Read the model definition and answer for the solid it produces. Units are mm, in the model's axes. A direction names the side the tool comes from. Give positions to 0.01 mm unless a question says otherwise; leave off trailing zeros. Loops run counter-clockwise (first coordinate to the right, second up) from the corner with the lowest first, then second, coordinate; pieces in that order, holes last. Notation, with made-up numbers: (-36.75, -24) -> (-31.75, -24) arc R29 ccw to (-31.75, 2) -> close; hole circle Ø6 at (41, 46.25). An arc over 180 degrees is marked (long way). One line per item, written item: value. Start each with the question number.
from build123d import *

# Parameters (mm, degrees)
F3_DEPTH = 13.97


with BuildPart() as f1:
    # F0 (on Front) → F1 (revolve)
    with BuildSketch(Plane.XZ):
        with BuildLine():
            Line((7.876178, -20.195216), (8.228687, 0))
            Line((8.228687, 0), (7.876178, 20.195216))
            ThreePointArc((7.876178, 20.195216), (7.838213, 20.283583), (7.749197, 20.32))
            Line((7.749197, 20.32), (6.347803, 20.32))
            ThreePointArc((6.347803, 20.32), (6.258787, 20.283583), (6.220822, 20.195216))
            Line((6.220822, 20.195216), (5.868313, 0))
            Line((5.868313, 0), (7.041552, -20.200364))
            ThreePointArc((7.041552, -20.200364), (7.081178, -20.285369), (7.168338, -20.32))
            Line((7.168338, -20.32), (7.749197, -20.32))
            ThreePointArc((7.749197, -20.32), (7.838213, -20.283583), (7.876178, -20.195216))
        make_face()
    revolve(axis=Axis((0, 0, 5.243593), (0, 0, -1)))

    # F2 (on Top) → F3 (join, symmetric)
    with BuildSketch(Plane.XY):
        with BuildLine():
            Line((-2.459506, 0.112758), (1.096672, 6.948127))
            ThreePointArc((1.096672, 6.948127), (0.550133, 7.015935), (0, 7.041552))
            Line((0, 7.041552), (-2.903674, 0.532035))
            Line((-2.903674, 0.532035), (-2.959069, 0.407848))
            ThreePointArc((-2.959069, 0.407848), (-2.841238, 0.036922), (-2.459506, 0.112758))
        make_face()
        with BuildLine():
            ThreePointArc((5.486935, -4.655437), (5.818928, -4.216025), (6.116179, -3.752404))
            Line((6.116179, -3.752404), (1.930609, 2.01701))
            Line((1.930609, 2.01701), (1.850757, 2.127077))
            ThreePointArc((1.850757, 2.127077), (1.470611, 2.210495), (1.345421, 1.841988))
            Line((1.345421, 1.841988), (5.486935, -4.655437))
        make_face()
        with BuildLine():
            Line((0.940514, -2.31779), (-6.757178, -2.655735))
            ThreePointArc((-6.757178, -2.655735), (-6.542632, -3.162955), (-6.28975, -3.652192))
            Line((-6.28975, -3.652192), (0.799493, -2.912089))
            Line((0.799493, -2.912089), (0.93474, -2.897969))
            ThreePointArc((0.93474, -2.897969), (1.197055, -2.610462), (0.940514, -2.31779))
        make_face()
    extrude(amount=F3_DEPTH, both=True)

    # F4 (on Front) → F5 (revolve, cut)
    with BuildSketch(Plane.XZ):
        Polygon((6.11216, 13.97), (0, 13.97), (0, 7.85784), align=None)
        Polygon((0, -7.290308), (0, -13.97), (6.679692, -13.97), align=None)
    revolve(axis=Axis((0, 0, 5.243593), (0, 0, -1)), mode=Mode.SUBTRACT)


solid = f1.part
Item 1: Section C-C, the plane z = 8.5 is taken. Determine the outline of the cut face in (x, y).
Item 2: For faces 4 (the conical face through (-2.26, -2.93, -10.99)), 5 (the flat face through (-4.6, 5.7, -20.32)), 6 (the conical face through (-1.93, -2.97, 11.4)), determine the directions among +Z, -Z, +X, -X, +Y, -Y from which every point of the face is accessible in a straight line to the end or side of a thin tool.
Item 3: Consider L1, parallel to Y at x = 1, z = -1; L2, parallel to X at y = 4.75, z = -1; L3, parallel to Y at x = -4.5, z = -9. Determine where each line is inside the solid, lowest interval first. Write a range as [from, to].
Item 4: Section A-A, the plane z = -1 is taken. Determine the outline of the cut face in (x, y), plus the area to 3 significant figures.
Item 5: Section B-B, the plane y = 4 is taken. State how many separate pieces and enclosed holes the cut face has, plus the area to 3 significant figures.
Item 6: Determine the mould class of faces 1 (the conical face through (-1.745, 7.859, 10.239)), 2 (the conical face through (3.211, -0.409, 11.094)), 3 (the flat face through (-3, 6, 20.32)) for opening direction Y: pulls with the +Y half, pulls with the -Y half, needs draft (parallel to the pull), parting line crosses it, or undercut.
Item 7: Flat-ended cylindrical pins translate along their axes: pin 1 (3 mm diameter, centred on x = 1, z = 1, fed in from -Y); pin 2 (6 mm diameter, centred on y = -4.5, z = -8, fed in from -X); pin 3 (4 mm diameter, centred on y = 0, z = 3, fed in from -X); pin 4 (6 mm diameter, centred on x = 5.5, z = -1.5, fed in from -Y). Find the tip coordinate at first contact, or state that the pin passes through.
Computed values:
1. outline: circle Ø16.16 at (0, 0); hole (-5.43, -2.6) -> (0.94, -2.32) arc R0.29 cw to (0.93, -2.9) -> (0.8, -2.91) -> (-4.89, -3.51) arc R6.02 ccw to (4.82, -3.6) -> (1.35, 1.84) arc R0.29 cw to (1.85, 2.13) -> (1.93, 2.02) -> (5.37, -2.72) arc R6.02 ccw to (0.6, 5.99) -> (-2.46, 0.11) arc R0.29 cw to (-2.96, 0.41) -> (-2.9, 0.53) -> (-0.47, 6) arc R6.02 ccw to start
2. face 4: -Z
2. face 5: -Z, +X, -X, +Y, -Y
2. face 6: +Z
3. L1: [-8.15, -5.84], [-2.88, -2.33], [5.84, 8.15]
3. L2: [-6.7, -3.54], [-1.02, -0.05], [3.54, 6.7]
3. L3: [-6.7, -4.54], [-3.47, -2.56], [4.54, 6.7]
4. outline: circle Ø16.42 at (0, 0); hole (-5.33, -2.59) -> (0.94, -2.32) arc R0.29 cw to (0.93, -2.9) -> (0.8, -2.91) -> (-4.79, -3.5) arc R5.93 ccw to (4.77, -3.52) -> (1.35, 1.84) arc R0.29 cw to (1.85, 2.13) -> (1.93, 2.02) -> (5.31, -2.64) arc R5.93 ccw to (0.55, 5.9) -> (-2.46, 0.11) arc R0.29 cw to (-2.96, 0.41) -> (-2.9, 0.53) -> (-0.51, 5.9) arc R5.93 ccw to start
4. area: 116 mm²
5. separate pieces: 3
5. enclosed holes: 0
5. area: 199 mm²
6. face 1: parting line crosses it
6. face 2: undercut
6. face 3: needs draft
7. pin 1: y = -8.23
7. pin 2: x = -7.95
7. pin 3: x = -8.21
7. pin 4: y = -7.81
